Input: dimensioned drawing with shaded views. Units: mm. Origin: part minimum x, y, z. Give positions to 0.01 mm unless a question says otherwise; leave off trailing zeros. Loops run counter-clockwise (first coordinate to the right, second up) from the corner with the lowest first, then second, coordinate; pieces in that order, holes last.
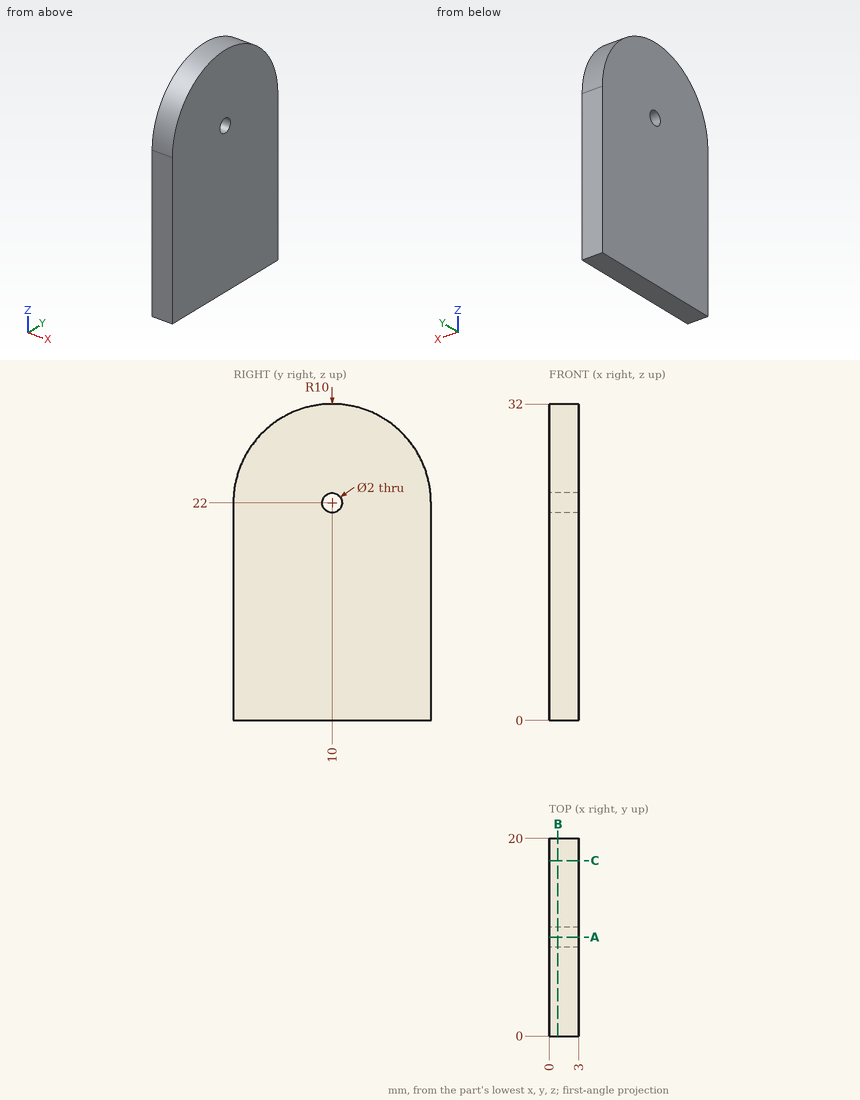
(1) Section C-C, the plane y = 17.75. Return the cut outline in (x, z), then the cut area to 3 significant figures.
A:
outline: (0, 0) - (3, 0) - (3, 28.32) - (0, 28.32) - close
area: 85.0 mm2
(2) Section A-A, the plane y = 10. Return the cut outline in (x, z), then the cut area to 3 significant figures.
A:
outline: (0, 0) - (3, 0) - (3, 21) - (0, 21) - close; (0, 23) - (3, 23) - (3, 32) - (0, 32) - close
area: 90.0 mm2
(3) Ray query, line 1 along Y through (x, z) = (1.45, 22); line 2 along Z through (x, y) = (0.95, 10); line 3 along Z through (x, y) = (0.2, 11.75). Return the intervals inside material, ascending.
A:
line 1: y = 0 to 9, 11 to 20
line 2: z = 0 to 21, 23 to 32
line 3: z = 0 to 31.85
(4) First-contact query: pin 1 (1.2 mm diameter, centred on y = 10, z = 22, fed in from -X). Flat tip, straight axial feed; report the tip coordinate or a pass-through.
A:
pin 1: passes through
(5) Section B-B, the plane x = 0.9. Return the cut outline in (y, z).
A:
outline: (0, 0) - (20, 0) - (20, 22) arc R10 ccw to (0, 22) - close; hole circle Ø2 at (10, 22)
